Source: CAD feature listing. Evaluate the final solid. Frame: model axes, mm. A direction names the side the tool comes from. Round coordinates to 2 decimals unless told otherwise and drop trailing zeros. Order: outer loops, then holes, each group sorted by start corner. A loop starts at its lowest first (then second) coordinate and runs counter-clockwise, first axis right, second up. Notation, with made-up numbers: (52.25, 73) - (77.25, 73) arc R19 cw to (77.25, 87) - close; hole circle Ø3 at (89, 29). An arc over 180 degrees is marked (long way). Return JSON: item names as keys, results as strings. Group by question number.
1) Ray query, line 1 (Y direction, x = -13.5, z = 1.75); line 2 (X direction, y = 47.5, z = 1.1); line 3 (Y direction, x = 1.5, z = 2). Return the intervals inside material, ascending. Write a range as from..to.
2) Access query for faces 1 (the flat face through (7, 51, 1)), 2 (the flat face through (0, 60, 1)). Directions: +Z, -Z, +X, -X, +Y, -Y. A direction counts if a zero-diameter tool reaches every point of the face in a straight line with its end or side. Return the directions, or none.
3) Section C-C, the plane y = 38.75. Return loops of the section in (x, z), plus the area to 3 significant figures.
4) Section B-B, the plane x = 13.5. Return loops of the section in (y, z).
5) Section A-A, the plane y = 35. Return loops of the section in (x, z).
6) Section D-D, the plane z = 2.45. Return loops of the section in (x, y).
7) Mould query, pull axis X, two halves, no side actions, for faces 3 (the flat face through (18.5, 45, 1)), 4 (the flat face through (0, 30, 2)), 5 (the cylindrical face through (-15.1, 55.07, 1.48)), 6 (the cylindrical face through (11.9, 55.07, 1.48)). Classes: pulls with the +X half, pulls with the -X half, needs draft (parallel to the pull), parting line crosses it, or undercut.
```python
from build123d import *

# Parameters (mm, degrees)
SKETCH_1_W          = 37
SKETCH_1_H          = 120
SKETCH_1_R          = 1.6
SKETCH_1_R_2        = 3
EXTRUDE_1_DEPTH     = 3
SKETCH_2_W          = 37
SKETCH_2_H          = 90
CUT_EXTRUDE_1_DEPTH = 3
SKETCH_3_W          = 17
SKETCH_3_H          = 15
CUT_EXTRUDE_2_DEPTH = 63.858969129
CHAMFER_1_SIZE      = 3


with BuildPart() as part:
    # ｽｹｯﾁ1 → ﾎﾞｽ - 押し出し1 (new body)
    # profile 1 of 2: a face of its own
    with BuildSketch(Plane.XY):
        Rectangle(SKETCH_1_W, SKETCH_1_H)
        with Locations((13.5, -55)):
            Circle(SKETCH_1_R, mode=Mode.SUBTRACT)
        with Locations((13.5, -35)):
            Circle(SKETCH_1_R_2, mode=Mode.SUBTRACT)
        with Locations((-13.5, -55)):
            Circle(SKETCH_1_R, mode=Mode.SUBTRACT)
        with Locations((-13.5, -35)):
            Circle(SKETCH_1_R_2, mode=Mode.SUBTRACT)
        with Locations((13.5, 35)):
            Circle(SKETCH_1_R, mode=Mode.SUBTRACT)
        with Locations((13.5, 55)):
            Circle(SKETCH_1_R, mode=Mode.SUBTRACT)
        with Locations((-13.5, 35)):
            Circle(SKETCH_1_R, mode=Mode.SUBTRACT)
        with Locations((-13.5, 55)):
            Circle(SKETCH_1_R, mode=Mode.SUBTRACT)
    # profile 2 of 2: a face of its own
    with BuildSketch(Plane.XY):
        Polygon((-18.5, -25), (-18.5, -60), (18.5, -60), (18.5, 60), (-18.5, 60), (-18.5, 25), align=None)
        with Locations((-13.5, -55)):
            Circle(SKETCH_1_R, mode=Mode.SUBTRACT)
        with Locations((-13.5, -35)):
            Circle(SKETCH_1_R_2, mode=Mode.SUBTRACT)
        with Locations((13.5, -55)):
            Circle(SKETCH_1_R, mode=Mode.SUBTRACT)
        with Locations((13.5, -35)):
            Circle(SKETCH_1_R_2, mode=Mode.SUBTRACT)
        with Locations((-13.5, 35)):
            Circle(SKETCH_1_R, mode=Mode.SUBTRACT)
        with Locations((-13.5, 55)):
            Circle(SKETCH_1_R, mode=Mode.SUBTRACT)
        with Locations((13.5, 35)):
            Circle(SKETCH_1_R, mode=Mode.SUBTRACT)
        with Locations((13.5, 55)):
            Circle(SKETCH_1_R, mode=Mode.SUBTRACT)
    extrude(amount=EXTRUDE_1_DEPTH)

    # ｽｹｯﾁ2 → ｶｯﾄ - 押し出し1 (cut)
    with BuildSketch(Plane.XY.offset(3)):
        with Locations((0, -15)):
            Rectangle(SKETCH_2_W, SKETCH_2_H)
    extrude(amount=-CUT_EXTRUDE_1_DEPTH, mode=Mode.SUBTRACT)

    # ｽｹｯﾁ3 → ｶｯﾄ - 押し出し2 (cut, through all)
    with BuildSketch(Plane(origin=(0, 0, 0), x_dir=(-1, 0, 0), z_dir=(0, 0, -1))):
        with Locations((0, 45)):
            Rectangle(SKETCH_3_W, SKETCH_3_H)
    extrude(amount=-CUT_EXTRUDE_2_DEPTH, mode=Mode.SUBTRACT)

    # 面取り1
    chamfer_1_edges = [part.edges().sort_by_distance(p)[0] for p in [
        (8.5, 37.5, 1.5),
        (8.5, 52.5, 1.5),
        (-8.5, 52.5, 1.5),
        (-8.5, 37.5, 1.5),
    ]]
    chamfer(chamfer_1_edges, length=CHAMFER_1_SIZE)


solid = part.part
```
Geometry check:
{
 "1": {"line 1": "30..33.4, 36.6..53.4, 56.6..60", "line 2": "-18.5..-8.5, 8.5..18.5", "line 3": "30..37.5, 52.5..60"},
 "2": {"face 1": "+Z, -Z", "face 2": "+Z, -Z, +X, -X, +Y"},
 "3": {"outline": "(-18.5, 0) - (-6.75, 0) - (-6.75, 3) - (-18.5, 3) - close; (6.75, 0) - (18.5, 0) - (18.5, 3) - (6.75, 3) - close", "area": "70.5 mm2"},
 "4": {"outline": "(30, 0) - (33.4, 0) - (33.4, 3) - (30, 3) - close; (36.6, 0) - (53.4, 0) - (53.4, 3) - (36.6, 3) - close; (56.6, 0) - (60, 0) - (60, 3) - (56.6, 3) - close"},
 "5": {"outline": "(-18.5, 0) - (-15.1, 0) - (-15.1, 3) - (-18.5, 3) - close; (-11.9, 0) - (11.9, 0) - (11.9, 3) - (-11.9, 3) - close; (15.1, 0) - (18.5, 0) - (18.5, 3) - (15.1, 3) - close"},
 "6": {"outline": "(-18.5, 30) - (18.5, 30) - (18.5, 60) - (-18.5, 60) - close; hole circle Ø3.2 at (-13.5, 35); hole circle Ø3.2 at (-13.5, 55); hole (-8.5, 40.5) - (-5.5, 37.5) - (5.5, 37.5) - (8.5, 40.5) - (8.5, 49.5) - (5.5, 52.5) - (-5.5, 52.5) - (-8.5, 49.5) - close; hole circle Ø3.2 at (13.5, 35); hole circle Ø3.2 at (13.5, 55)"},
 "7": {"face 3": "pulls with the +X half", "face 4": "needs draft", "face 5": "undercut", "face 6": "undercut"}
}
